```python
from build123d import *

# Parameters (mm, degrees)
BOSS_EXTRU_1_DEPTH      = 3
ESQUISSE4_W             = 10
ESQUISSE4_H             = 2.8
ENL_V_MAT_EXTRU_2_DEPTH = 114.176852757
ESQUISSE5_W             = 2.8
ESQUISSE5_H             = 10
ENL_V_MAT_EXTRU_3_DEPTH = 114.176852757
ESQUISSE6_W             = 40
ESQUISSE6_H             = 20
ENL_V_MAT_EXTRU_4_DEPTH = 114.176852757
ESQUISSE7_R             = 2
ENL_V_MAT_EXTRU_5_DEPTH = 114.176852757


with BuildPart() as part:
    # Esquisse2 → Boss.-Extru.1 (new body)
    with BuildSketch(Plane.XY):
        with BuildLine():
            Line((10, 0), (70, 0))
            ThreePointArc((70, 0), (77.071067812, 2.928932188), (80, 10))
            Line((80, 10), (80, 70))
            ThreePointArc((80, 70), (77.071067812, 77.071067812), (70, 80))
            Line((70, 80), (10, 80))
            ThreePointArc((10, 80), (2.928932188, 77.071067812), (0, 70))
            Line((0, 70), (0, 10))
            ThreePointArc((0, 10), (2.928932188, 2.928932188), (10, 0))
        make_face()
    extrude(amount=BOSS_EXTRU_1_DEPTH)

    # Esquisse4 → Enlèv. mat.-Extru.2 (cut, through all)
    with BuildSketch(Plane.XY.offset(3)):
        with Locations((60, 73.6)):
            Rectangle(ESQUISSE4_W, ESQUISSE4_H)
        with Locations((20, 73.6)):
            Rectangle(ESQUISSE4_W, ESQUISSE4_H)
        with Locations((20, 6.6)):
            Rectangle(ESQUISSE4_W, ESQUISSE4_H)
        with Locations((60, 6.6)):
            Rectangle(ESQUISSE4_W, ESQUISSE4_H)
    extrude(amount=-ENL_V_MAT_EXTRU_2_DEPTH, mode=Mode.SUBTRACT)

    # Esquisse5 → Enlèv. mat.-Extru.3 (cut, through all)
    with BuildSketch(Plane.XY.offset(3)):
        with Locations((73.6, 60)):
            Rectangle(ESQUISSE5_W, ESQUISSE5_H)
        with Locations((6.4, 60)):
            Rectangle(ESQUISSE5_W, ESQUISSE5_H)
        with Locations((6.4, 20)):
            Rectangle(ESQUISSE5_W, ESQUISSE5_H)
        with Locations((73.6, 20)):
            Rectangle(ESQUISSE5_W, ESQUISSE5_H)
    extrude(amount=-ENL_V_MAT_EXTRU_3_DEPTH, mode=Mode.SUBTRACT)

    # Esquisse6 → Enlèv. mat.-Extru.4 (cut, through all)
    with BuildSketch(Plane.XY.offset(3)):
        with Locations((40, 40)):
            Rectangle(ESQUISSE6_W, ESQUISSE6_H)
    extrude(amount=-ENL_V_MAT_EXTRU_4_DEPTH, mode=Mode.SUBTRACT)

    # Esquisse7 → Enlèv. mat.-Extru.5 (cut, through all)
    with BuildSketch(Plane(origin=(0, 0, 0), x_dir=(-1, 0, 0), z_dir=(0, 0, -1))):
        with Locations((-15, 34.5)):
            Circle(ESQUISSE7_R)
        with Locations((-15, 44.5)):
            Circle(ESQUISSE7_R)
        with Locations((-64, 34.5)):
            Circle(ESQUISSE7_R)
        with Locations((-64, 44.5)):
            Circle(ESQUISSE7_R)
    extrude(amount=-ENL_V_MAT_EXTRU_5_DEPTH, mode=Mode.SUBTRACT)


solid = part.part
```
For this review, take the finished solid that the model builds, in its own axes (mm). A direction names the side the tool comes from. Give positions to 0.01 mm unless a question says otherwise; leave off trailing zeros. Order: outer loops, then holes, each group sorted by start corner. A loop starts at its lowest first (then second) coordinate and runs counter-clockwise, first axis right, second up.
1) Wall thickness on line 1 (X direction, y = 17, z = 1.35); line 2 (Y direction, x = 64, z = 1.6); line 3 (X direction, y = 48, z = 0.7): over which ranges is each line inside the solid? List them lowest first.
2) Take a section at C-C (x = 64). Give the boundary of the cut face in (y, z).
3) For faces 4 (the face through (3.01, 77.15, 1.48)), 5 (the face through (20, 40, 2)), list the 3-axis set-ups (+Z, -Z, +X, -X, +Y, -Y) from which the entire face can be reached by the end or side of a thin tool; tool diameter is ignored.
4) Take a section at D-D (y = 21.5). Give the boundary of the cut face in (x, z).
5) The part is to be moulded in two halves that separate along Y. For faces 1 (the face through (77.15, 76.99, 1.48)), 2 (the face through (2.85, 3.01, 1.48)), 3 (the face through (7.8, 20, 2)), say which applies: released by +Y, released by -Y, zero draft, split by the parting line, or undercut.
6) Insertion check: pin 1 (0.8 mm diameter, centred on y = 73.5, z = 2, fed in from -X); pin 2 (0.8 mm diameter, centred on x = 74, z = 1.5, fed in from +Y); pin 3 (1.4 mm diameter, centred on y = 7, z = 2, fed in from +X). Each pin has a flat end and moves straight along its axis. Give the tip position at first contact, or say it passes through.
7) Take a section at B-B (y = 34.5). Give the boundary of the cut face in (x, z), then the cut area to 3 significant figures.
8) Take a section at A-A (x = 40). Give the boundary of the cut face in (y, z), then the cut area to 3 significant figures.
Derived:
1. line 1: x = 0 to 5, 7.8 to 72.2, 75 to 80
1. line 2: y = 0 to 5.2, 8 to 32.5, 36.5 to 42.5, 46.5 to 72.2, 75 to 80
1. line 3: x = 0 to 20, 60 to 80
2. outline: (0, 0) - (5.2, 0) - (5.2, 3) - (0, 3) - close; (8, 0) - (32.5, 0) - (32.5, 3) - (8, 3) - close; (36.5, 0) - (42.5, 0) - (42.5, 3) - (36.5, 3) - close; (46.5, 0) - (72.2, 0) - (72.2, 3) - (46.5, 3) - close; (75, 0) - (80, 0) - (80, 3) - (75, 3) - close
3. face 4: +Z, -Z, -X, +Y
3. face 5: +Z, -Z
4. outline: (0, 0) - (5, 0) - (5, 3) - (0, 3) - close; (7.8, 0) - (72.2, 0) - (72.2, 3) - (7.8, 3) - close; (75, 0) - (80, 0) - (80, 3) - (75, 3) - close
5. face 1: released by +Y
5. face 2: released by -Y
5. face 3: undercut
6. pin 1: stops at x = 0.49
6. pin 2: stops at y = 79.33
6. pin 3: stops at x = 79.73
7. outline: (0, 0) - (13, 0) - (13, 3) - (0, 3) - close; (17, 0) - (20, 0) - (20, 3) - (17, 3) - close; (60, 0) - (62, 0) - (62, 3) - (60, 3) - close; (66, 0) - (80, 0) - (80, 3) - (66, 3) - close
7. area: 96.0 mm2
8. outline: (0, 0) - (30, 0) - (30, 3) - (0, 3) - close; (50, 0) - (80, 0) - (80, 3) - (50, 3) - close
8. area: 180 mm2
